Autodesk Inventor part; units mm, degrees
ref_plane "YZ Plane" through (0, 0, 0) normal (1, 0, 0) x (0, 1, 0)
ref_plane "XZ Plane" through (0, 0, 0) normal (0, 1, 0) x (-1, 0, 0)
ref_plane "XY Plane" through (0, 0, 0) normal (0, 0, 1) x (1, 0, 0)
sketch "Sketch1" plane through (0, 0, 0) normal (0, 0, 1) x (1, 0, 0)
  line L0 (0, 0) -> (0, 50.8)
  line L1 (0, 0) -> (50.8, 0)
  line L2 (3.175, 50.8) -> (3.175, 3.175)
  line L3 (3.175, 3.175) -> (50.8, 3.175)
  line L4 (0, 50.8) -> (3.175, 50.8)
  line L5 (50.8, 3.175) -> (50.8, 0)
  dimension "d0" = 50.8
  dimension "d1" = 50.8
  dimension "d2" = 3.175
extrude "Extrusion1" add sketch "Sketch1" along normal blind 1016
sketch "Sketch2" plane through (3.175, 3.175, 0) normal (0, 1, 0) x (1, 0, 0)
  line L0 (-3.175, 0) -> (-3.175, -1016)
  line L1 (47.625, -1016) -> (-3.175, -1016)
  line L2 (-3.175, -1016) -> (-3.175, -990.6)
  line L3 (-3.175, -990.6) -> (47.625, -990.6)
  line L4 (47.625, -990.6) -> (47.625, -1016)
  line L5 (0, 0) -> (0, -1016)
  line L6 (47.625, 0) -> (47.625, -1016)
  line L7 (0, -990.6) -> (47.625, -990.6)
  line L8 (47.625, -990.6) -> (47.625, -830.58)
  line L9 (47.625, -830.58) -> (0, -830.58)
  line L10 (0, -830.58) -> (0, -990.6)
  line L11 (47.625, 0) -> (0, 0)
  line L12 (0, 0) -> (0, -25.4)
  line L13 (0, -25.4) -> (47.625, -25.4)
  line L14 (47.625, -25.4) -> (47.625, 0)
  line L15 (47.625, -25.4) -> (0, -25.4)
  line L16 (0, -25.4) -> (0, -185.42)
  line L17 (0, -185.42) -> (47.625, -185.42)
  line L18 (47.625, -185.42) -> (47.625, -25.4)
  dimension "d5" = 25.4
  dimension "d6" = 160.02
  dimension "d7" = 25.4
  dimension "d8" = 160.02
extrude "Extrusion2" cut sketch "Sketch2" against normal blind 1016 contours L5 L9 L6 L3 | L5 L13 L6 L17
sketch "Sketch5" plane through (3.175, 3.175, 185.42) normal (0, 1, 0) x (1, 0, 0)
  line L0 (47.625, 0) -> (47.625, -645.16)
  line L1 (0, 0) -> (47.625, 0)
  line L2 (47.625, 0) -> (47.625, -50.8)
  line L3 (47.625, -50.8) -> (0, -50.8)
  line L4 (0, -50.8) -> (0, 0)
  line L5 (0, 0) -> (0, -645.16)
  line L6 (47.625, -645.16) -> (0, -645.16)
  line L7 (0, -645.16) -> (0, -594.36)
  line L8 (0, -594.36) -> (47.625, -594.36)
  line L9 (47.625, -594.36) -> (47.625, -645.16)
  point P0 (-3.175, 185.42)
  dimension "d21" = 50.8
  dimension "d22" = 50.8
extrude "Extrusion4" cut sketch "Sketch5" against normal blind 1016 contours L0 L3 L4 L1 | L0 L6 L5 L8
sketch "Sketch6" plane through (3.175, 3.175, 0) normal (1, 0, 0) x (0, 0, -1)
  circle A0 centre (-152.4, -101.6) radius 114.3
  circle A1 centre (-863.6, -101.6) radius 114.3
  point P0 (0, -3.175)
  dimension "d25" = 228.6
extrude "Extrusion5" cut sketch "Sketch6" against normal blind 1016
sketch "Sketch7" plane through (3.175, 3.175, 1016) normal (0, 1, 0) x (1, 0, 0)
  line L0 (0, 990.6) -> (0, 921.712)
  line L1 (47.625, 990.6) -> (0, 990.6)
  line L2 (0, 990.6) -> (0, 939.8)
  line L3 (0, 939.8) -> (47.625, 939.8)
  line L4 (47.625, 939.8) -> (47.625, 990.6)
  line L5 (0, 94.288) -> (0, 25.4)
  line L6 (47.625, 24.8924) -> (0, 24.8924)
  line L7 (0, 24.8924) -> (0, 75.6924)
  line L8 (0, 75.6924) -> (47.625, 75.6924)
  line L9 (47.625, 75.6924) -> (47.625, 24.8924)
  point P0 (-3.175, 1016)
  dimension "d28" = 50.8
  dimension "d29" = 50.8
extrude "Extrusion6" add sketch "Sketch7" against normal blind 3.175
sketch "Sketch8" plane through (3.175, 3.175, 0) normal (1, 0, 0) x (0, 0, -1)
  line L0 (0, 47.625) -> (-1016, 47.625)
  line L1 (-26.088, 47.625) -> (2.2813, 19.2557)
  line L2 (-26.088, 47.625) -> (14.0323, 47.625) construction
  line L3 (2.2813, 19.2557) -> (0, 47.625)
  line L4 (0, 47.625) -> (-26.088, 47.625)
  point P0 (0, -3.175)
  dimension "d32" = 45
extrude "Extrusion7" cut sketch "Sketch8" against normal blind 3.175
sketch "Sketch9" plane through (3.175, 3.175, 1016) normal (1, 0, 0) x (0, 0, -1)
  line L0 (989.912, 47.625) -> (0, 47.625)
  line L1 (330.2, 47.625) -> (330.2, -3.175)
  point P0 (1016, -3.175)
  point P1 (330.2, 23.8125)
  point P2 (838.2, 22.225)
  point P3 (711.2, 22.225)
  point P4 (584.2, 22.225)
  point P5 (457.2, 22.225)
hole "Hole2" at (3.175, 25.4, 177.8) at (3.175, 25.4, 304.8) at (3.175, 25.4, 431.8) at (3.175, 25.4, 558.8) direction (-1, 0, 0) diameter 9.525 end through all
sketch "Sketch10" plane through (3.175, 3.175, 1016) normal (0, 1, 0) x (1, 0, 0)
  line L0 (0, 75.6924) -> (43.0144, 32.678)
  line L1 (0, 75.6924) -> (60.8315, 75.6924) construction
  line L2 (43.0144, 32.678) -> (47.625, 28.0674)
  line L3 (47.625, 75.6924) -> (47.625, 0)
  line L4 (47.625, 75.6924) -> (0, 75.6924)
  line L5 (0, 94.288) -> (0, 75.6924)
  line L6 (0, 236.22) -> (70.4888, 306.7088)
  line L7 (0, 236.22) -> (99.6862, 236.22) construction
  line L8 (70.4888, 306.7088) -> (70.4888, 236.22)
  line L9 (70.4888, 236.22) -> (0, 236.22)
  line L10 (0, 779.78) -> (0, 236.22)
  line L11 (0, 779.78) -> (47.625, 732.155)
  line L12 (47.625, 732.155) -> (47.625, 779.78)
  line L13 (47.625, 779.78) -> (47.625, 236.22)
  line L14 (47.625, 779.78) -> (0, 779.78)
  line L15 (0, 939.8) -> (47.625, 987.425)
  line L16 (47.625, 1016) -> (47.625, 939.8)
  line L17 (47.625, 939.8) -> (0, 939.8)
  point P0 (-3.175, 1016)
  dimension "d42" = 45
  dimension "d43" = 45
extrude "Extrusion8" cut sketch "Sketch10" against normal blind 25.4 contours L4 L3 L2 L0 | L6 L13 L9 | L6 L8 L9 L13 | L14 L12 L11 | L15 L16 L17
sketch "Sketch11" plane through (3.175, 3.175, 1016) normal (1, 0, 0) x (0, 0, -1)
  line L0 (989.912, 47.625) -> (0, 47.625)
  line L1 (330.2, 47.625) -> (332.5489, 47.625)
  line L2 (332.5489, 47.625) -> (332.5489, 61.5215)
  line L3 (332.5489, 61.5215) -> (330.2, 61.5215)
  line L4 (330.2, 61.5215) -> (330.2, 47.625)
  point P0 (1016, -3.175)
extrude "Extrusion9" add sketch "Sketch11" against normal blind 254
properties part number "Conveyor Support"
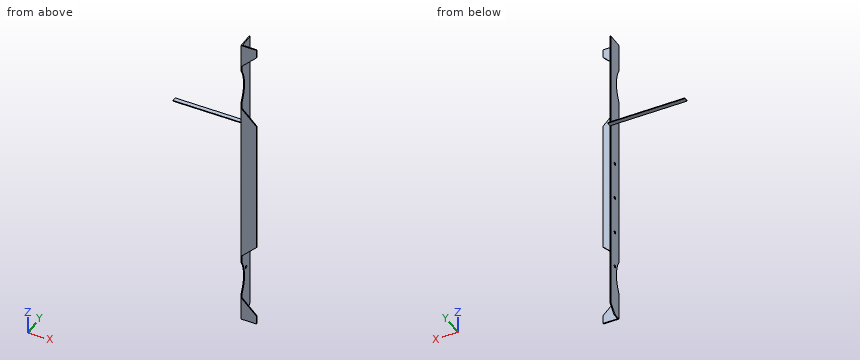
The listing builds one solid part. Answer for the finished solid, in the listing's coordinates (mm). Round coordinates to 2 decimals unless told otherwise and drop trailing zeros. Order: outer loops, then holes, each group sorted by start corner. A loop starts at its lowest first (then second) coordinate and runs counter-clockwise, first axis right, second up. Notation, with made-up numbers: (36, 39) -> (73, 39) arc R12 ccw to (73, 56) -> close; hole circle Ø9 at (19, -23). An arc over 180 degrees is marked (long way). Write each question's results on one line, items separated by ' | '. Start each with the question number.
Q1. Find section A-A (z = 513). Determine the outline of the cut face in (x, y) (3 decimals).
Q2. Find section D-D (z = 104.5). Determine the outline of the cut face in (x, y) (3 decimals).
Q3. Straight lines are drawn through the part: probe 1 along Z at (x, y) = (1.2, 25.4); probe 2 along Y at (x, z) = (1, 431); probe 3 along Z at (x, y) = (1, 25). For each, find the intervals that lie inside material, in ascending order. Write a range as from..to.
Q4. Each of these flat-tipped pins is pushed along its axis until it touches: pin 1 (4 mm diameter, centred on x = -1, z = 658.5, fed in from +Y); pin 2 (4 mm diameter, centred on x = -165.5, y = 61, fed in from -Z); pin 3 (11 mm diameter, centred on x = -106.5, y = 55, fed in from +Z). Where does it stop, or does it pass through?
Q5. Find section B-B (x = -77). Determine the outline of the cut face in (y, z).
Q6. Find section C-C (z = 768). Determine the outline of the cut face in (x, y) (3 decimals).
Worked answers:
1) outline: (0, 0) -> (50.8, 0) -> (50.8, 3.175) -> (3.175, 3.175) -> (3.175, 50.8) -> (0, 50.8) -> close
2) outline: (0, 5.354) -> (3.175, 5.354) -> (3.175, 50.8) -> (0, 50.8) -> close
3) probe 1: z = 0.69..173.04, 182.56..300.04, 309.56..427.04, 436.56..554.04, 563.56..1016 | probe 2: y = 0..20.71, 30.09..50.8 | probe 3: z = 0.29..173.05, 182.55..300.05, 309.55..427.05, 436.55..554.05, 563.55..1016
4) pin 1: stops at y = 50.8 | pin 2: stops at z = 683.45 | pin 3: stops at z = 685.8
5) outline: (50.8, 683.45) -> (64.7, 683.45) -> (64.7, 685.8) -> (50.8, 685.8) -> close
6) outline: (0, 0) -> (14.955, 0) -> (14.955, 3.175) -> (3.175, 3.175) -> (3.175, 50.8) -> (0, 50.8) -> close
